from build123d import *

# Parameters (mm, degrees)
BOSS_EXTRUDE1_DEPTH = 22
SKETCH2_R           = 1.25
CUT_EXTRUDE1_DEPTH  = 16
CUT_EXTRUDE2_REACH  = 64.643
SKETCH3_W           = 12
SKETCH3_H           = 14.2
SKETCH4_W           = 7
SKETCH4_H           = 5
BOSS_EXTRUDE2_DEPTH = 1
CIRPATTERN1_COUNT   = 2
CUT_EXTRUDE3_REACH  = 46.934
SKETCH5_R           = 3.5
SKETCH5_R_2         = 2.3


with BuildPart() as part:
    # Sketch1 → Boss-Extrude1 (new, symmetric)
    with BuildSketch(Plane.XY):
        Polygon((-18.2, 0), (18.2, 0), (18.2, 30), (25.2, 30), (25.2, -6), (-25.2, -6), (-25.2, 30), (-18.2, 30), align=None)
    extrude(amount=BOSS_EXTRUDE1_DEPTH, both=True)

    # Sketch2 → Cut-Extrude1 (cut)
    with BuildSketch(Plane(origin=(0, 30, 0), x_dir=(1, 0, 0), z_dir=(0, 1, 0))):
        with Locations(Location((-21.1, -3.6, 0), (0, 0, 270))):
            Circle(SKETCH2_R)
        with Locations(Location((-21.1, 3.6, 0), (0, 0, 90))):
            Circle(SKETCH2_R)
        with Locations(Location((21.1, 3.6, 0), (0, 0, 270))):
            Circle(SKETCH2_R)
        with Locations(Location((21.1, -3.6, 0), (0, 0, 90))):
            Circle(SKETCH2_R)
    extrude(amount=-CUT_EXTRUDE1_DEPTH, mode=Mode.SUBTRACT)

    # Sketch3 → Cut-Extrude2 (cut, up to next)
    with BuildSketch(Plane(origin=(25.2, 0, 0), x_dir=(0, 0, -1), z_dir=(1, 0, 0)), mode=Mode.PRIVATE) as cut_extrude2_sk1:
        with Locations((-16, 22.9)):
            Rectangle(SKETCH3_W, SKETCH3_H)
    cut_extrude2_tool1 = extrude(cut_extrude2_sk1.sketch, amount=-CUT_EXTRUDE2_REACH, mode=Mode.PRIVATE) & part.part
    # Sketch3 → Cut-Extrude2 (cut, up to next)
    with BuildSketch(Plane(origin=(25.2, 0, 0), x_dir=(0, 0, -1), z_dir=(1, 0, 0)), mode=Mode.PRIVATE) as cut_extrude2_sk2:
        Polygon((-10, 15.8), (-22, 15.8), (-22, 10.8), (4, 10.8), (4, 15.8), align=None)
    cut_extrude2_tool2 = extrude(cut_extrude2_sk2.sketch, amount=-CUT_EXTRUDE2_REACH, mode=Mode.PRIVATE) & part.part
    cut_extrude2_1 = cut_extrude2_tool1.solids().sort_by_distance((25.2, 22.9, 16))[0]
    add(cut_extrude2_1, mode=Mode.SUBTRACT)
    cut_extrude2_2 = cut_extrude2_tool2.solids().sort_by_distance((25.2, 13.3, 9))[0]
    add(cut_extrude2_2, mode=Mode.SUBTRACT)
    cut_extrude2 = cut_extrude2_1 + cut_extrude2_2  # Cut-Extrude2 as one shape, for the pattern or mirror that repeats it

    # Sketch4 → Boss-Extrude2 (add)
    with BuildSketch(Plane.XY.offset(10)):
        with Locations((21.7, 13.3)):
            Rectangle(SKETCH4_W, SKETCH4_H)
    boss_extrude2 = extrude(amount=-BOSS_EXTRUDE2_DEPTH)

    # CirPattern1: Cut-Extrude2, Boss-Extrude2 ×2 about axis
    cirpattern1_axis = Axis((0, -7.8, 0), (0, 1, 0))
    add([cut_extrude2.rotate(cirpattern1_axis, i * 360 / CIRPATTERN1_COUNT) for i in range(1, CIRPATTERN1_COUNT)], mode=Mode.SUBTRACT)
    add([boss_extrude2.rotate(cirpattern1_axis, i * 360 / CIRPATTERN1_COUNT) for i in range(1, CIRPATTERN1_COUNT)])

    # Sketch5 → Cut-Extrude3 (cut, up to next)
    with BuildSketch(Plane(origin=(0, 0, 0), x_dir=(1, 0, 0), z_dir=(0, 1, 0)), mode=Mode.PRIVATE) as cut_extrude3_sk1:
        with Locations(Location((0, 0, 0), (0, 0, 270))):
            Circle(SKETCH5_R)
    cut_extrude3_tool1 = extrude(cut_extrude3_sk1.sketch, amount=-CUT_EXTRUDE3_REACH, mode=Mode.PRIVATE) & part.part
    # Sketch5 → Cut-Extrude3 (cut, up to next)
    with BuildSketch(Plane(origin=(0, 0, 0), x_dir=(1, 0, 0), z_dir=(0, 1, 0)), mode=Mode.PRIVATE) as cut_extrude3_sk2:
        with Locations(Location((-11, 11, 0), (0, 0, 270))):
            Circle(SKETCH5_R_2)
    cut_extrude3_tool2 = extrude(cut_extrude3_sk2.sketch, amount=-CUT_EXTRUDE3_REACH, mode=Mode.PRIVATE) & part.part
    # Sketch5 → Cut-Extrude3 (cut, up to next)
    with BuildSketch(Plane(origin=(0, 0, 0), x_dir=(1, 0, 0), z_dir=(0, 1, 0)), mode=Mode.PRIVATE) as cut_extrude3_sk3:
        with Locations(Location((11, 11, 0), (0, 0, 270))):
            Circle(SKETCH5_R_2)
    cut_extrude3_tool3 = extrude(cut_extrude3_sk3.sketch, amount=-CUT_EXTRUDE3_REACH, mode=Mode.PRIVATE) & part.part
    # Sketch5 → Cut-Extrude3 (cut, up to next)
    with BuildSketch(Plane(origin=(0, 0, 0), x_dir=(1, 0, 0), z_dir=(0, 1, 0)), mode=Mode.PRIVATE) as cut_extrude3_sk4:
        with Locations(Location((11, -11, 0), (0, 0, 270))):
            Circle(SKETCH5_R_2)
    cut_extrude3_tool4 = extrude(cut_extrude3_sk4.sketch, amount=-CUT_EXTRUDE3_REACH, mode=Mode.PRIVATE) & part.part
    # Sketch5 → Cut-Extrude3 (cut, up to next)
    with BuildSketch(Plane(origin=(0, 0, 0), x_dir=(1, 0, 0), z_dir=(0, 1, 0)), mode=Mode.PRIVATE) as cut_extrude3_sk5:
        with Locations(Location((-11, -11, 0), (0, 0, 270))):
            Circle(SKETCH5_R_2)
    cut_extrude3_tool5 = extrude(cut_extrude3_sk5.sketch, amount=-CUT_EXTRUDE3_REACH, mode=Mode.PRIVATE) & part.part
    add(cut_extrude3_tool1.solids().sort_by_distance((0, 0, 0))[0], mode=Mode.SUBTRACT)
    add(cut_extrude3_tool2.solids().sort_by_distance((-11, 0, -11))[0], mode=Mode.SUBTRACT)
    add(cut_extrude3_tool3.solids().sort_by_distance((11, 0, -11))[0], mode=Mode.SUBTRACT)
    add(cut_extrude3_tool4.solids().sort_by_distance((11, 0, 11))[0], mode=Mode.SUBTRACT)
    add(cut_extrude3_tool5.solids().sort_by_distance((-11, 0, 11))[0], mode=Mode.SUBTRACT)


solid = part.part
Input: part model. Units: mm. Frame: model coordinates. A direction names the side the tool comes from. Give positions to 0.01 mm unless a question says otherwise; leave off trailing zeros. Order: outer loops, then holes, each group sorted by start corner. A loop starts at its lowest first (then second) coordinate and runs counter-clockwise, first axis right, second up.
Q1. Section B-B on x = 0. Output: boundary loops of the cut face in (y, z), and give its area (3 significant figures).
Checked values:
outline: (-6, -22) - (0, -22) - (0, -3.5) - (-6, -3.5) - close; (-6, 3.5) - (0, 3.5) - (0, 22) - (-6, 22) - close
area: 222 mm2
Q2. Ray query, probe 1 along Z at (x, y) = (21.1, 25.5); probe 2 along X at (y, z) = (23, -3.6); probe 3 along X at (y, z) = (-3.5, -11). Return the intervals inside material, ascending.
Checked values:
probe 1: z = -22 to -4.85, -2.35 to 2.35, 4.85 to 10
probe 2: x = -25.2 to -22.35, -19.85 to -18.2, 18.2 to 19.85, 22.35 to 25.2
probe 3: x = -25.2 to -13.3, -8.7 to 8.7, 13.3 to 25.2
Q3. Section D-D on y = 10. Output: boundary loops of the cut face in (x, z).
Checked values:
outline: (-25.2, -22) - (-18.2, -22) - (-18.2, 22) - (-25.2, 22) - close; (18.2, -22) - (25.2, -22) - (25.2, 22) - (18.2, 22) - close
Q4. Contact query for flat-ended pins moving along their axis: pin 1 Ø1 at (y, z) = (18, -15) entering from -X; pin 2 Ø1.5 at (x, z) = (7, -10.5) entering from +Y; pin 3 Ø5.5 at (x, z) = (-21.5, -4.5) entering from +Y; pin 4 Ø7.5 at (x, z) = (-20, -18.5) entering from +Y. Output: stop coordinate, or through.
Checked values:
pin 1: stops at x = 18.2
pin 2: stops at y = 0
pin 3: stops at y = 30
pin 4: stops at y = 10.8
Q5. Set-up query: faces 4 (the flat face through (22, 21, 10)), 5 (the flat face through (-22, 10.8, -3)), 6 (the cylindrical face through (-21.579, 22.112, 4.755)). Return all of +Z, -Z, +X, -X, +Y, -Y with unobstructed straight access to the full face (end or side cutting, diameter ignored); none if empty.
Checked values:
face 4: +Z, +X, +Y
face 5: -X
face 6: +Y
Q6. Draft query along Y for faces 1 (the flat face through (22, 13, -4)), 2 (the flat face through (22, 30, -6)), 3 (the cylindrical face through (-22.154, 22.999, -4.272)). Return one class per face: +Y half, -Y half, draft (parallel to the pull), parting line (faces both ways), or undercut.
Checked values:
face 1: undercut
face 2: +Y half
face 3: draft
Q7. Section C-C on z = -8. Output: boundary loops of the cut face in (x, y).
Checked values:
outline: (-25.2, -6) - (25.2, -6) - (25.2, 30) - (18.2, 30) - (18.2, 0) - (-18.2, 0) - (-18.2, 10.8) - (-25.2, 10.8) - close; (-25.2, 15.8) - (-18.2, 15.8) - (-18.2, 30) - (-25.2, 30) - close
Q8. Section A-A on y = 23.5. Output: boundary loops of the cut face in (x, z), and give its area (3 significant figures).
Checked values:
outline: (-25.2, -10) - (-18.2, -10) - (-18.2, 22) - (-25.2, 22) - close; (18.2, -22) - (25.2, -22) - (25.2, 10) - (18.2, 10) - close; hole circle Ø2.5 at (-21.1, -3.6); hole circle Ø2.5 at (-21.1, 3.6); hole circle Ø2.5 at (21.1, -3.6); hole circle Ø2.5 at (21.1, 3.6)
area: 428 mm2
